from build123d import *

# Parameters (mm, degrees)
F0_W     = 145
F0_H     = 37.25
F0_R     = 12.5
F1_DEPTH = 3
F2_W     = 60
F2_H     = 30
F3_DEPTH = 17
F4_W     = 7
F4_H     = 5
F5_DEPTH = 2
F6_R     = 2
F7_W     = 20.5
F7_H     = 17
F8_DEPTH = 4


with BuildPart() as f1:
    # F0 (on Front) → F1 (new body)
    with BuildSketch(Plane.XZ):
        Rectangle(F0_W, F0_H)
        with Locations((-52.5, -0.375)):
            Circle(F0_R, mode=Mode.SUBTRACT)
        with Locations((52.5, -0.375)):
            Circle(F0_R, mode=Mode.SUBTRACT)
    extrude(amount=F1_DEPTH)

    # F2 (on face) → F3 (join)
    with BuildSketch(Plane.XZ.offset(3)):
        with Locations((0, -3.625)):
            Rectangle(F2_W, F2_H)
    extrude(amount=F3_DEPTH)

    # F4 (on face) → F5 (cut)
    with BuildSketch(Plane.XY.offset(11.375)):
        with Locations((-17.5, -13)):
            Rectangle(F4_W, F4_H)
        with Locations((17.5, -13)):
            Rectangle(F4_W, F4_H)
    extrude(amount=-F5_DEPTH, mode=Mode.SUBTRACT)

    # F6
    f6_edges = [f1.edges().sort_by_distance(p)[0] for p in [
        (0, -3, 11.375),
        (30, -3, -3.625),
        (-30, -3, -3.625),
        (-30, -20, -3.625),
        (0, -20, 11.375),
        (30, -20, -3.625),
    ]]
    fillet(f6_edges, radius=F6_R)

    # F7 (on face) → F8 (cut)
    with BuildSketch(Plane.XZ.offset(20)):
        with Locations((0, -10.125)):
            Rectangle(F7_W, F7_H)
    extrude(amount=-F8_DEPTH, mode=Mode.SUBTRACT)


solid = f1.part
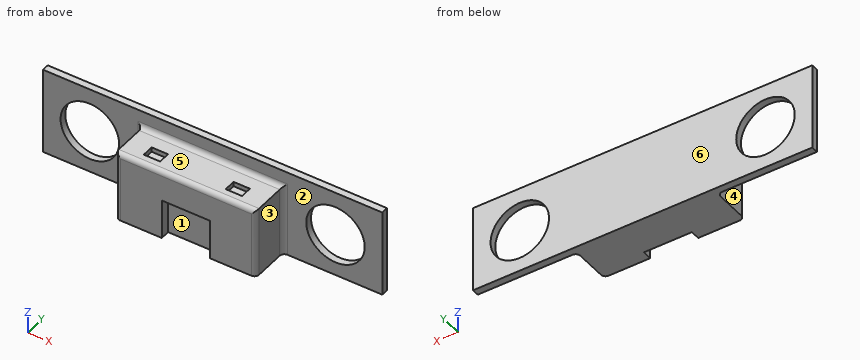
Build history of the part. All positions in model axes, mm. Face numbers are marked on the shaded views. A direction names the side the tool comes from. Round coordinates to 2 decimals unless told otherwise and drop trailing zeros. Write each loop counter-clockwise with the first axis right and the second up, starting at its lowest first coordinate (ties: lowest second). Pieces come first, ordered by that corner, then holes. Notation, with made-up numbers: M 8.5,33.5 L 40.5,33.5 A32 ccw 40.5,69.5 Z; hole C 21.5,44 d9. An arc over 180 degrees is marked long. Answer as a JSON object with one key per item and string values. Group by question number.
(1) Flat gauge pins, fed straight in: pin 1 (5 mm diameter, centred on y = -16, z = -6, fed in from -X); pin 2 (1.5 mm diameter, centred on x = -17, y = -13, fed in from +Z) (3 decimals); pin 3 (6.5 mm diameter, centred on y = -8.5, z = -8, fed in from +X); pin 4 (6 mm diameter, centred on x = 40, y = -7, fed in from -Z). Where does each tip first touch, or does it go through?
(2) Cut at D-D (x = -26.5). Give the cut face in (y, z) (3 decimals), and give its area (3 significant figures).
(3) Cut at B-B (z = 2.5). Give the cut face in (x, y).
(4) Mould opens along X. For the marked faces 1, 2 and 3 say: pulls with the +X half, pulls with the -X half, needs draft (parallel to the pull), parting line crosses it, or undercut.
(5) Which spindle directions (+Z, -Z, +X, -X, +Y, -Y) get a long thin tool onto all of the face, cutting with end or side? Do the marked faces 4, 5 and 6. Say none if no direction does.
(6) Cut at C-C (z = -14.5). Give the cut face in (x, y), and give its area (3 significant figures).
(7) Cut at A-A (x = 52.5). Give the cut face in (y, z) (3 decimals).
(8) Drill centre lines: L1, parallel to Z at x = 52.5, y = -2.3 (3 decimals); L2, parallel to X at y = -1.25, z = 4; L3, parallel to X at y = -2.5, z = -10.5. Where is each one in solid material? Low to high.
Responses:
{
 "1": {"pin 1": "stops at x = -30", "pin 2": "stops at z = 9.375", "pin 3": "stops at x = 30", "pin 4": "passes through"},
 "2": {"outline": "M -20,-18.625 L 0,-18.625 L 0,18.625 L -3,18.625 L -3,13.375 A2 cw -5,11.375 L -18,11.375 A2 ccw -20,9.375 Z", "area": "622 mm2"},
 "3": {"outline": "M -72.5,-3 L -64.66,-3 L -64.66,0 L -72.5,0 Z; M -40.34,-3 L -32,-3 A2 cw -30,-5 L -30,-18 A2 ccw -28,-20 L 28,-20 A2 ccw 30,-18 L 30,-5 A2 cw 32,-3 L 40.34,-3 L 40.34,0 L -40.34,0 Z; M 64.66,-3 L 72.5,-3 L 72.5,0 L 64.66,0 Z"},
 "4": {"face 1": "undercut", "face 2": "needs draft", "face 3": "pulls with the +X half"},
 "5": {"face 4": "+Z, -Z, -X, -Y", "face 5": "+Z, +X, -X, -Y", "face 6": "+Z, -Z, +X, -X, +Y"},
 "6": {"outline": "M -72.5,-3 L -32,-3 A2 cw -30,-5 L -30,-18 A2 ccw -28,-20 L -10.25,-20 L -10.25,-16 L 10.25,-16 L 10.25,-20 L 28,-20 A2 ccw 30,-18 L 30,-5 A2 cw 32,-3 L 72.5,-3 L 72.5,0 L -72.5,0 Z", "area": "1,370 mm2"},
 "7": {"outline": "M -3,-18.625 L 0,-18.625 L 0,-12.875 L -3,-12.875 Z; M -3,12.125 L 0,12.125 L 0,18.625 L -3,18.625 Z"},
 "8": {"L1": "z = -18.625 to -12.875, 12.125 to 18.625", "L2": "x = -72.5 to -64.21, -40.79 to 40.79, 64.21 to 72.5", "L3": "x = -72.5 to -59.83, -45.17 to 45.17, 59.83 to 72.5"}
}
